Geometry check sheet. Reference: the model listing, model coordinates, mm. Coordinates: 2 decimals unless noted, no trailing zeros. Loops run counter-clockwise (first coordinate to the right, second up) from the corner with the lowest first, then second, coordinate; pieces in that order, holes last. Notation, with made-up numbers: M -5.5,66 L 0.5,66 A25 cw 0.5,103 Z; hole C 46,-20 d9. An arc over 180 degrees is marked long. Use CSV: the item, a comma, the result in double quotes.
```python
from build123d import *

# Parameters (mm, degrees)
F2_DEPTH = 12.7


with BuildPart() as f2:
    # F0 (on Top) → F2 (new body)
    with BuildSketch(Plane.XY):
        with BuildLine():
            ThreePointArc((-229.577515, -84.918341), (-234.665402, -90.006231), (-234.665401, -97.201592))
            ThreePointArc((-234.665401, -97.201592), (-229.577512, -102.289481), (-222.38215, -102.289481))
            Line((-222.38215, -102.289481), (-159.00424, -76.037492))
            ThreePointArc((-159.00424, -76.037492), (-89.802561, -89.802561), (-76.037492, -159.00424))
            Line((-76.037492, -159.00424), (-102.289483, -222.382153))
            ThreePointArc((-102.289483, -222.382153), (-102.289481, -229.577513), (-97.201592, -234.665401))
            ThreePointArc((-97.201592, -234.665401), (-90.00623, -234.665401), (-84.91834, -229.577512))
            Line((-84.91834, -229.577512), (-58.66635, -166.199602))
            ThreePointArc((-58.66635, -166.199602), (0, -127), (58.66635, -166.199602))
            Line((58.66635, -166.199602), (84.918341, -229.577515))
            ThreePointArc((84.918341, -229.577515), (90.006231, -234.665402), (97.201592, -234.665401))
            ThreePointArc((97.201592, -234.665401), (102.289481, -229.577512), (102.289481, -222.38215))
            Line((102.289481, -222.38215), (76.037492, -159.00424))
            ThreePointArc((76.037492, -159.00424), (89.802561, -89.802561), (159.00424, -76.037492))
            Line((159.00424, -76.037492), (222.382153, -102.289483))
            ThreePointArc((222.382153, -102.289483), (229.577514, -102.289481), (234.665401, -97.201591))
            ThreePointArc((234.665401, -97.201591), (234.665401, -90.006229), (229.577512, -84.91834))
            Line((229.577512, -84.91834), (166.199602, -58.66635))
            ThreePointArc((166.199602, -58.66635), (127, 0), (166.199602, 58.66635))
            Line((166.199602, 58.66635), (229.577515, 84.918341))
            ThreePointArc((229.577515, 84.918341), (234.665402, 90.006231), (234.665401, 97.201592))
            ThreePointArc((234.665401, 97.201592), (229.577512, 102.289481), (222.38215, 102.289481))
            Line((222.38215, 102.289481), (159.00424, 76.037492))
            ThreePointArc((159.00424, 76.037492), (89.802561, 89.802561), (76.037492, 159.00424))
            Line((76.037492, 159.00424), (102.289483, 222.382153))
            ThreePointArc((102.289483, 222.382153), (102.289481, 229.577514), (97.201591, 234.665401))
            ThreePointArc((97.201591, 234.665401), (90.006229, 234.665401), (84.91834, 229.577512))
            Line((84.91834, 229.577512), (58.66635, 166.199602))
            ThreePointArc((58.66635, 166.199602), (0, 127), (-58.66635, 166.199602))
            Line((-58.66635, 166.199602), (-84.918341, 229.577515))
            ThreePointArc((-84.918341, 229.577515), (-90.006232, 234.665402), (-97.201593, 234.665401))
            ThreePointArc((-97.201593, 234.665401), (-102.289481, 229.577511), (-102.289481, 222.38215))
            Line((-102.289481, 222.38215), (-76.037492, 159.00424))
            ThreePointArc((-76.037492, 159.00424), (-89.802561, 89.802561), (-159.00424, 76.037492))
            Line((-159.00424, 76.037492), (-222.382153, 102.289483))
            ThreePointArc((-222.382153, 102.289483), (-229.577514, 102.289481), (-234.665401, 97.201591))
            ThreePointArc((-234.665401, 97.201591), (-234.665401, 90.006229), (-229.577512, 84.91834))
            Line((-229.577512, 84.91834), (-166.199602, 58.66635))
            ThreePointArc((-166.199602, 58.66635), (-127, 0), (-166.199602, -58.66635))
            Line((-166.199602, -58.66635), (-229.577515, -84.918341))
        make_face()
    extrude(amount=F2_DEPTH)


solid = f2.part
```
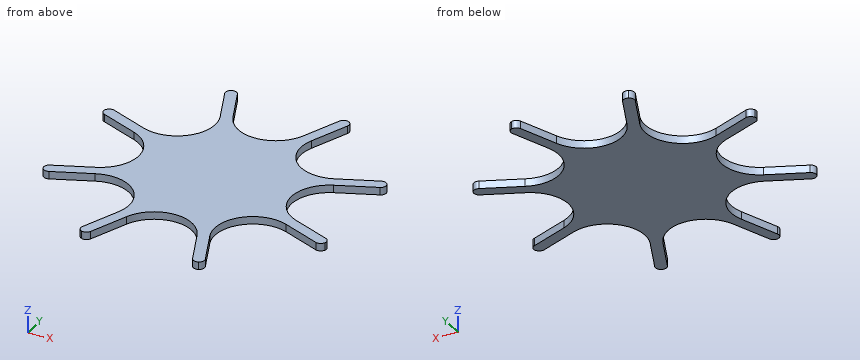
1. Section check C-C, the plane y = -16.5. Record the cut outline in (x, z), plus the area to 3 significant figures.
The answers:
outline,"M -129.18,0 L 129.18,0 L 129.18,12.7 L -129.18,12.7 Z"
area,"3,280 mm^2"
2. Thickness scan on line 1 (Y direction, x = 89, z = 7.5); line 2 (X direction, y = 97, z = 12); line 3 (Y direction, x = -135, z = 10.5). Record the ranges inside material, lowest first. Write a range as [from, to].
The answers:
line 1,"[-234.18, -190.3], [-90.62, 90.62], [190.3, 234.18]"
line 2,"[-234.75, -209.61], [-83.61, 83.61], [209.61, 234.75]"
line 3,"[-71.2, -30.85], [30.85, 71.2]"
3. Section check B-B, the plane x = 204.5. Record the cut outline in (y, z).
The answers:
outline,"M -94.88,0 L -74.53,0 L -74.53,12.7 L -94.88,12.7 Z; M 74.53,0 L 94.88,0 L 94.88,12.7 L 74.53,12.7 Z"
4. Gauge pin test, flat ends, axial feed: P1, Ø2, axis at x = 33.5, z = 7.5, coming from the +Y side; P2, Ø3, axis at x = 188, z = 6.5, coming from the -Y side; P3, Ø3, axis at x = 25, z = 10, coming from the -Y side. Record the tip position at first contact, or that the pin passes through.
The answers:
P1,"y = 137.19"
P2,"y = -88.67"
P3,"y = -132.79"
5. Section check A-A, the plane y = 185. Record the cut outline in (x, z).
The answers:
outline,"M -86.81,0 L -66.45,0 L -66.45,12.7 L -86.81,12.7 Z; M 66.45,0 L 86.81,0 L 86.81,12.7 L 66.45,12.7 Z"
6. Section check D-D, the plane x = 117. Record the cut outline in (y, z), plus the area to 3 significant figures.
The answers:
outline,"M -73.72,0 L 73.72,0 L 73.72,12.7 L -73.72,12.7 Z"
area,"1,870 mm^2"
